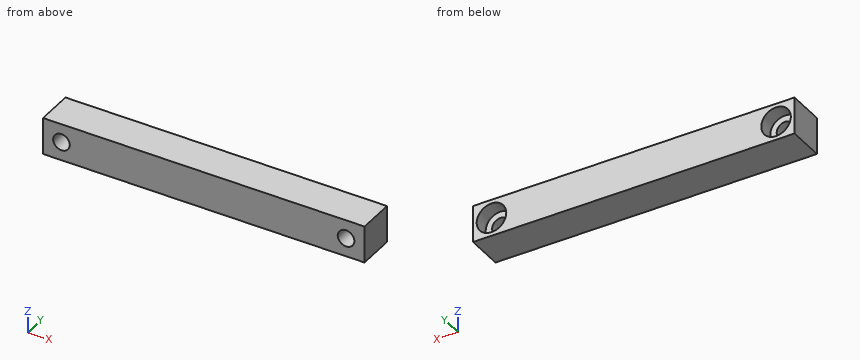
```python
from build123d import *

# Parameters (mm, degrees)
SKETCH1_W                      = 87
SKETCH1_H                      = 10
BOSS_EXTRUDE1_DEPTH            = 10
CBORE_FOR_M4_SHCS2_D           = 4.5
CBORE_FOR_M4_SHCS2_CBORE_D     = 8
CBORE_FOR_M4_SHCS2_CBORE_DEPTH = 4


with BuildPart() as part:
    # Sketch1 → Boss-Extrude1 (new body)
    with BuildSketch(Plane(origin=(0, 0, 0), x_dir=(1, 0, 0), z_dir=(0, 1, 0))):
        Rectangle(SKETCH1_W, SKETCH1_H)
    extrude(amount=BOSS_EXTRUDE1_DEPTH)

    # CBORE for M4 SHCS2 (through all)
    with Locations(Plane(origin=(0, 10, 0), x_dir=(1, 0, 0), z_dir=(0, 1, 0))):
        with Locations((-38.5, 0)):
            cbore_for_m4_shcs2 = CounterBoreHole(CBORE_FOR_M4_SHCS2_D / 2, CBORE_FOR_M4_SHCS2_CBORE_D / 2, CBORE_FOR_M4_SHCS2_CBORE_DEPTH)

    # Mirror3: CBORE for M4 SHCS2 across plane
    add(cbore_for_m4_shcs2.mirror(Plane(origin=(0, 0, 0), x_dir=(0, 0, 1), z_dir=(1, 0, 0))), mode=Mode.SUBTRACT)


solid = part.part
```
For this review, take the finished solid that the model builds, in its own axes (mm). Give positions to 0.01 mm unless a question says otherwise; leave off trailing zeros. Write each loop counter-clockwise with the first axis right and the second up, starting at its lowest first coordinate (ties: lowest second). Pieces come first, ordered by that corner, then holes. Notation, with made-up numbers: M 5,57.5 L 49,57.5 A26 ccw 49,86.5 Z; hole C 12.5,45 d11. An arc over 180 degrees is marked long. One line per item, written item: value.
1) Take a section at D-D, the plane x = 37. Write out the cut boundary in (y, z).
Results are:
outline: M 0,-5 L 10,-5 L 10,-3.71 L 6,-3.71 L 6,-1.68 L 0,-1.68 Z; M 0,1.68 L 6,1.68 L 6,3.71 L 10,3.71 L 10,5 L 0,5 Z
2) Take a section at A-A, the plane x = -38.5. Write out the cut boundary in (y, z), then the cut area to 3 significant figures.
Results are:
outline: M 0,-5 L 10,-5 L 10,-4 L 6,-4 L 6,-2.25 L 0,-2.25 Z; M 0,2.25 L 6,2.25 L 6,4 L 10,4 L 10,5 L 0,5 Z
area: 41.0 mm²
3) For line 1 (Z direction, x = -38.5, y = 9.2); line 2 (X direction, y = 6.25, z = -0.25); line 3 (X direction, y = 2, z = 2), list the stretches that pass through material, from the lowest coordinate up. Write a range as from..to.
Results are:
line 1: z = -5..-4, 4..5
line 2: x = -43.5..-42.49, -34.51..34.51, 42.49..43.5
line 3: x = -43.5..-39.53, -37.47..37.47, 39.53..43.5
4) Take a section at C-C, the plane y = 4.75. Write out the cut boundary in (x, z), then the cut area to 3 significant figures.
Results are:
outline: M -43.5,-5 L 43.5,-5 L 43.5,5 L -43.5,5 Z; hole C -38.5,0 d4.5; hole C 38.5,0 d4.5
area: 838 mm²
5) Take a section at B-B, the plane z = 0. Write out the cut boundary in (x, y), then the cut area to 3 significant figures.
Results are:
outline: M -43.5,0 L -40.75,0 L -40.75,6 L -42.5,6 L -42.5,10 L -43.5,10 Z; M -36.25,0 L 36.25,0 L 36.25,6 L 34.5,6 L 34.5,10 L -34.5,10 L -34.5,6 L -36.25,6 Z; M 40.75,0 L 43.5,0 L 43.5,10 L 42.5,10 L 42.5,6 L 40.75,6 Z
area: 752 mm²
